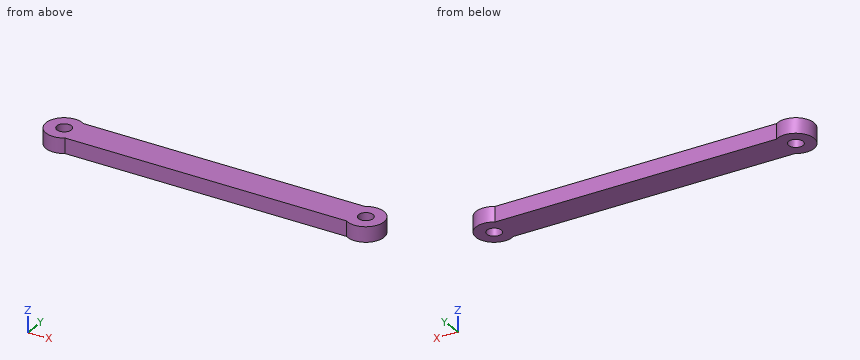
```python
from build123d import *

# Parameters (mm, degrees)
SKETCH14_R          = 1.2
BOSS_EXTRUDE1_DEPTH = 2.5
SKETCH15_R          = 3
SKETCH15_R_2        = 1.2
BOSS_EXTRUDE2_DEPTH = 2.5


with BuildPart() as part:
    # Sketch14 → Boss-Extrude1 (new body)
    with BuildSketch(Plane.XY):
        with BuildLine():
            Line((50, 2.5), (0, 2.5))
            ThreePointArc((0, 2.5), (-2.5, 0), (0, -2.5))
            Line((0, -2.5), (50, -2.5))
            ThreePointArc((50, -2.5), (52.5, 0), (50, 2.5))
        make_face()
        Circle(SKETCH14_R, mode=Mode.SUBTRACT)
        with Locations((50, 0)):
            Circle(SKETCH14_R, mode=Mode.SUBTRACT)
    extrude(amount=BOSS_EXTRUDE1_DEPTH)

    # Sketch15 → Boss-Extrude2 (add)
    with BuildSketch(Plane.XY.offset(2.5)):
        with Locations((50, 0)):
            Circle(SKETCH15_R)
        with Locations((50, 0)):
            Circle(SKETCH15_R_2, mode=Mode.SUBTRACT)
        Circle(SKETCH15_R)
        Circle(SKETCH15_R_2, mode=Mode.SUBTRACT)
    extrude(amount=-BOSS_EXTRUDE2_DEPTH)


solid = part.part
```
Geometry check sheet. Reference: the model listing, model coordinates, mm. Give positions to 0.01 mm unless a question says otherwise; leave off trailing zeros. Write each loop counter-clockwise with the first axis right and the second up, starting at its lowest first coordinate (ties: lowest second). Pieces come first, ordered by that corner, then holes. Notation, with made-up numbers: (24, -39.75) -> (49, -39.75) arc R25 cw to (49, -3.75) -> close; hole circle Ø6 at (-1, 78). An arc over 180 degrees is marked (long way). Use one line per item in the form item = value.
Item 1: Sectioned sample at C-C on z = 1.95. Enter the section's corners in (x, y).
Results list:
outline = (1.66, -2.5) -> (48.34, -2.5) arc R3 ccw (long way) to (48.34, 2.5) -> (1.66, 2.5) arc R3 ccw (long way) to start; hole circle Ø2.4 at (0, 0); hole circle Ø2.4 at (50, 0)
Item 2: Depth check by flat-ended pin: pin 1 Ø3 at (x, y) = (0, 0) entering from +Z; pin 2 Ø2 at (x, y) = (50, 0) entering from -Z; pin 3 Ø0.8 at (x, z) = (19.5, 1.5) entering from +Y. Enter the tip coordinate at first touch or a pass-through.
Results list:
pin_1 = 2.5
pin_2 = through
pin_3 = 2.5
Item 3: Sectioned sample at B-B on y = 0. Enter the section's corners in (x, z), plus the area to 3 significant figures.
Results list:
outline = (-3, 0) -> (-1.2, 0) -> (-1.2, 2.5) -> (-3, 2.5) -> close; (1.2, 0) -> (48.8, 0) -> (48.8, 2.5) -> (1.2, 2.5) -> close; (51.2, 0) -> (53, 0) -> (53, 2.5) -> (51.2, 2.5) -> close
area = 128 mm2
Item 4: Sectioned sample at D-D on x = 30.5. Enter the section's corners in (y, z).
Results list:
outline = (-2.5, 0) -> (2.5, 0) -> (2.5, 2.5) -> (-2.5, 2.5) -> close
Item 5: Scan lines: line 1 (Y direction, x = 47, z = 0.45); line 2 (X direction, y = 0.8, z = 1.25); line 3 (X direction, y = 0.45, z = 2). Record each from-to range of solid material in increasing order.
Results list:
line_1 = -2.5 to 2.5
line_2 = -2.89 to -0.89, 0.89 to 49.11, 50.89 to 52.89
line_3 = -2.97 to -1.11, 1.11 to 48.89, 51.11 to 52.97
Item 6: Sectioned sample at A-A on x = 50. Enter the section's corners in (y, z), plus the area to 3 significant figures.
Results list:
outline = (-3, 0) -> (-1.2, 0) -> (-1.2, 2.5) -> (-3, 2.5) -> close; (1.2, 0) -> (3, 0) -> (3, 2.5) -> (1.2, 2.5) -> close
area = 9.00 mm2
